from build123d import *

# Parameters (mm, degrees)
BOX021_W          = 10
BOX021_H          = 10
BOX021_DEPTH      = 10
BOX004_W          = 10
BOX004_H          = 110
BOX004_DEPTH      = 10
CYLINDER004_R     = 3.5
CYLINDER004_DEPTH = 10
BOX002_W          = 1.5
BOX002_H          = 170
BOX002_DEPTH      = 30


with BuildPart() as reset:
    # Box021 → Box021 (new body)
    with BuildSketch(Plane(origin=(-2, 154, 7), x_dir=(1, 0, 0), z_dir=(0, 0, 1))):
        with Locations((5, 5)):
            Rectangle(BOX021_W, BOX021_H)
    extrude(amount=BOX021_DEPTH)


with BuildPart() as cube003:
    # Box004 → Box004 (new body)
    with BuildSketch(Plane(origin=(-3, 38, -5), x_dir=(1, 0, 0), z_dir=(0, 0, 1))):
        with Locations((5, 55)):
            Rectangle(BOX004_W, BOX004_H)
    extrude(amount=BOX004_DEPTH)


with BuildPart() as pwrjack:
    # Cylinder004 → Cylinder004 (new body)
    with BuildSketch(Plane(origin=(-3, 16, 7), x_dir=(0, 0, -1), z_dir=(1, 0, 0))):
        Circle(CYLINDER004_R)
    extrude(amount=CYLINDER004_DEPTH)


with BuildPart() as cut006:
    # Box002 → Box002 (new body)
    with BuildSketch(Plane.XY.offset(-10)):
        with Locations((0.75, 85)):
            Rectangle(BOX002_W, BOX002_H)
    extrude(amount=BOX002_DEPTH)

    # Cut003: cut pwrjack
    add(pwrjack.part, mode=Mode.SUBTRACT)

    # Cut: cut Cube003
    add(cube003.part, mode=Mode.SUBTRACT)

    # Cut006: cut reset
    add(reset.part, mode=Mode.SUBTRACT)


solid = cut006.part
Read the model definition and answer for the solid it produces. Units are mm, in the model's axes. Coordinates: 2 decimals unless noted, no trailing zeros. Write each loop counter-clockwise with the first axis right and the second up, starting at its lowest first coordinate (ties: lowest second). Pieces come first, ordered by that corner, then holes. Notation, with made-up numbers: (44, 3.5) -> (97, 3.5) arc R28 ccw to (97, 23.5) -> close; hole circle Ø3 at (40, 62.25). An arc over 180 degrees is marked (long way). Return JSON: item names as keys, results as strings.
(1) For a pull along Z with two mould halves and no side action, classify faces 1 (the cylindrical face through (0.74, 18.365, 9.58)), 2 (the flat face through (1.5, 84, 8)) as pulls with the +Z half, pulls with the -Z half, needs draft (parallel to the pull), parting line crosses it, or undercut.
Answers below:
{"face 1": "undercut", "face 2": "needs draft"}
(2) Consider line 1 along Z through (x, y) = (1, 124); line 2 along Y through (x, z) = (1.15, 3); line 3 along Y through (x, z) = (0.25, 7.75). Determine where each line is inside the solid, lowest interval first. Write a range as from..to.
Answers below:
{"line 1": "-10..-5, 5..20", "line 2": "0..38, 148..170", "line 3": "0..12.58, 19.42..154, 164..170"}
(3) This flat-tipped pin is pushed along its axis until it touches: P1, Ø5.5, axis at y = 16, z = 7, coming from the -X side. Where does it stop, or does it pass through?
Answers below:
{"P1": "through"}
(4) The part is cut by section A-A on x = 0.35. Give the vertices of the cut face in (y, z).
Answers below:
{"outline": "(0, -10) -> (170, -10) -> (170, 20) -> (0, 20) -> close; hole circle Ø7 at (16, 7); hole (38, -5) -> (148, -5) -> (148, 5) -> (38, 5) -> close; hole (154, 7) -> (164, 7) -> (164, 17) -> (154, 17) -> close"}
(5) The part is cut by section B-B on z = 2. Give the vertices of the cut face in (x, y).
Answers below:
{"outline": "(0, 0) -> (1.5, 0) -> (1.5, 38) -> (0, 38) -> close; (0, 148) -> (1.5, 148) -> (1.5, 170) -> (0, 170) -> close"}
(6) The part is cut by section C-C on y = 100.5. Give the vertices of the cut face in (x, z).
Answers below:
{"outline": "(0, -10) -> (1.5, -10) -> (1.5, -5) -> (0, -5) -> close; (0, 5) -> (1.5, 5) -> (1.5, 20) -> (0, 20) -> close"}
